Verification items for this drawing (mm, ordinates from the low corner). A direction names the side the tool comes from. Give positions to 0.01 mm unless a question says otherwise; leave off trailing zeros. Loops run counter-clockwise (first coordinate to the right, second up) from the corner with the lowest first, then second, coordinate; pieces in that order, holes last. Notation, with made-up numbers: M -37,81.25 L -17,81.25 A26 ccw -17,112.25 Z; hole C 61,41 d5. An arc over 180 degrees is marked long. Answer in a Markdown table with one row per item.
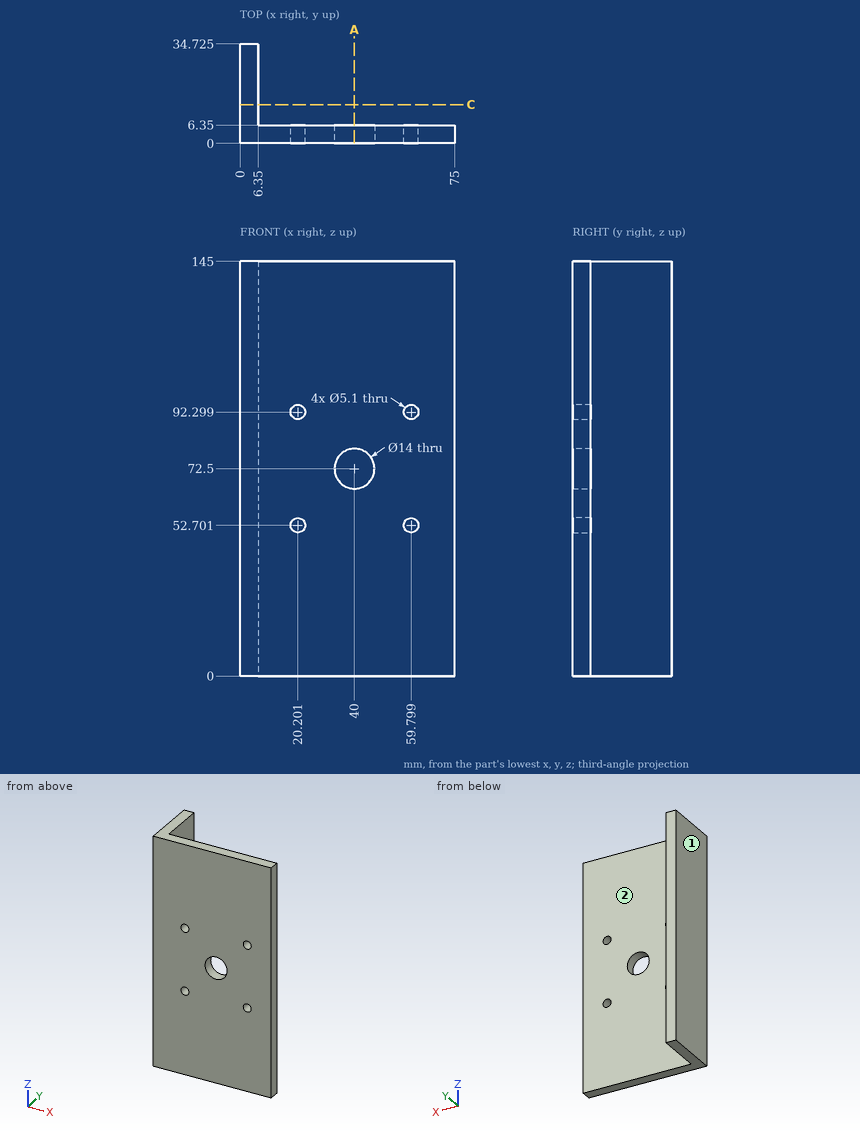
Item 1: Sectioned sample at A-A (x = 40). Record the cut outline in (y, z).
Reported:
| item | result |
|---|---|
| outline | M 0,0 L 6.35,0 L 6.35,65.5 L 0,65.5 Z; M 0,79.5 L 6.35,79.5 L 6.35,145 L 0,145 Z |
Item 2: Tool access check on the marked faces 1 and 2. Record the directions out of +Z, -Z, +X, -X, +Y, -Y that give a thin tool (end or side, any length) a straight path to the whole face; none if there is none.
Reported:
| item | result |
|---|---|
| face 1 | +Z, -Z, -X, +Y, -Y |
| face 2 | +Z, -Z, +X, +Y |
Item 3: Sectioned sample at C-C (y = 13.5). Record the cut outline in (x, z).
Reported:
| item | result |
|---|---|
| outline | M 0,0 L 6.35,0 L 6.35,145 L 0,145 Z |
Item 4: Go/stop test with flat-tipped pins: pin 1 (1.5 mm diameter, centred on y = 26.5, z = 108.5, fed in from +X); pin 2 (1 mm diameter, centred on x = 27, z = 41.5, fed in from +Y); pin 3 (4 mm diameter, centred on x = 59.8, z = 52.7, fed in from -Y). Record where each tip stops, or that it passes through.
Reported:
| item | result |
|---|---|
| pin 1 | stops at x = 6.35 |
| pin 2 | stops at y = 6.35 |
| pin 3 | passes through |
Item 5: Scan lines: L1, parallel to X at y = 3.5, z = 72.5; L2, parallel to X at y = 13, z = 128. Record each from-to range of solid material in increasing order. Write a range as [from, to].
Reported:
| item | result |
|---|---|
| L1 | x = [0, 33], [47, 75] |
| L2 | x = [0, 6.35] |
